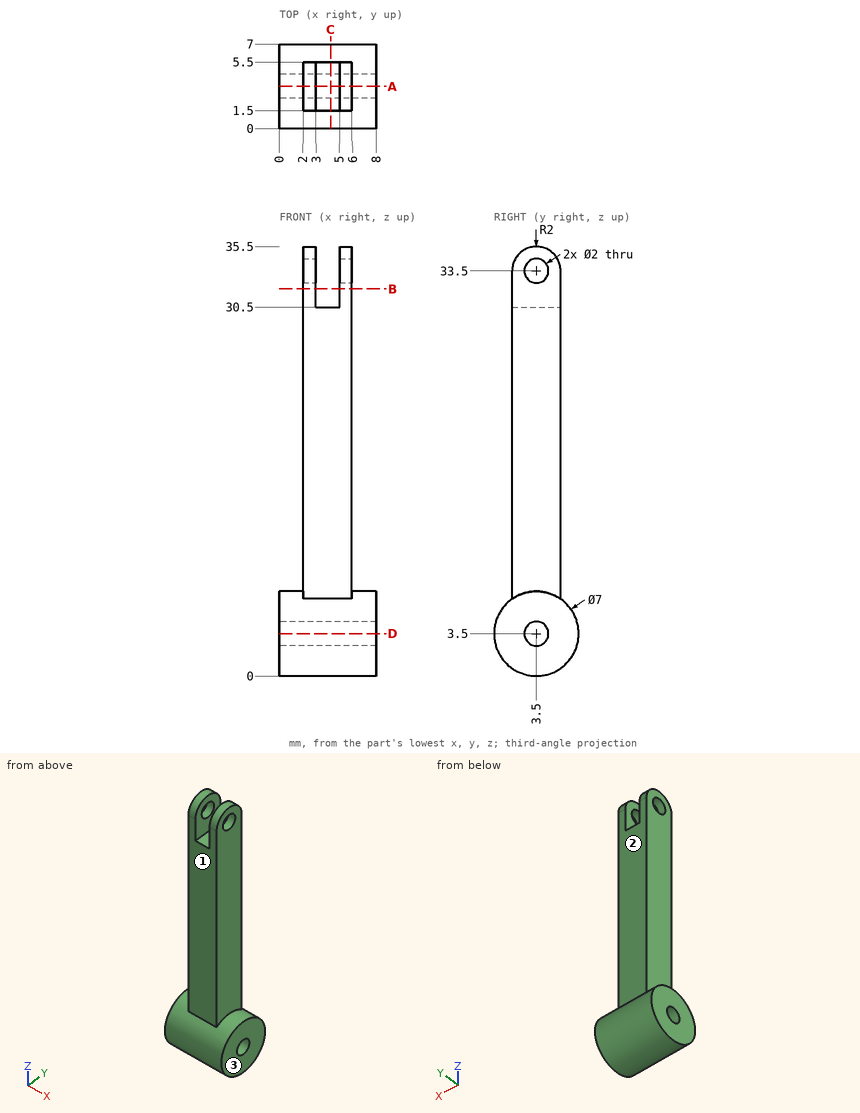
Study the drawing (mm; zero at the part's minimum x, y, z) and answer. A direction names the side the tool comes from. Give positions to 0.01 mm unless a question says otherwise; leave off trailing zeros. Write each loop counter-clockwise with the first axis right and the second up, starting at its lowest first coordinate (ties: lowest second). Pieces come first, ordered by that corner, then holes. Notation, with made-up numbers: (42, 1.25) -> (100, 1.25) arc R10 cw to (100, 20.25) -> close; hole circle Ø5 at (22, 38.5). An arc over 180 degrees is marked (long way). Write item = value, one per line.
Q1. Section B-B on z = 32 is taken. Determine the outline of the cut face in (x, y).
Computed values:
outline = (2, 1.5) -> (3, 1.5) -> (3, 5.5) -> (2, 5.5) -> close; (5, 1.5) -> (6, 1.5) -> (6, 5.5) -> (5, 5.5) -> close
Q2. Section C-C on x = 4.25 is taken. Determine the outline of the cut face in (y, z), and give its area (3 significant figures).
Computed values:
outline = (1.5, 6.37) arc R3.5 ccw (long way) to (5.5, 6.37) -> (5.5, 30.5) -> (1.5, 30.5) -> close; hole circle Ø2 at (3.5, 3.5)
area = 130 mm^2
Q3. Flat-ended cylindrical pins translate along their axes: pin 1 Ø1.8 at (y, z) = (3.5, 3.5) entering from +X; pin 2 Ø3 at (y, z) = (3, 27) entering from -X; pin 3 Ø3 at (x, z) = (5.5, 21.5) entering from -Y; pin 4 Ø4.5 at (x, z) = (3, 19) entering from +Y. Find the tip coordinate at first contact, or state that the pin passes through.
Computed values:
pin_1 = through
pin_2 = 2
pin_3 = 1.5
pin_4 = 5.5
Q4. Section D-D on z = 3.5 is taken. Determine the outline of the cut face in (x, y), and give its area (3 significant figures).
Computed values:
outline = (0, 0) -> (8, 0) -> (8, 2.5) -> (0, 2.5) -> close; (0, 4.5) -> (8, 4.5) -> (8, 7) -> (0, 7) -> close
area = 40.0 mm^2
Q5. Consider line 1 along Z through (x, y) = (5.55, 3.5); line 2 along Z through (x, y) = (4.75, 3.5); line 3 along X through (y, z) = (3, 9). Determine where each line is inside the solid, lowest interval first.
Computed values:
line_1 = 0 to 2.5, 4.5 to 32.5, 34.5 to 35.5
line_2 = 0 to 2.5, 4.5 to 30.5
line_3 = 2 to 6
Q6. A tool of negligible diameter and unlimited length cuts with its end or side. For the marked faces 1, 2 and 3, from which of +Z, -Z, +X, -X, +Y, -Y can it reach the whole face along a straight path? Write none if from no direction.
Computed values:
face_1 = +Z, +X, -X, -Y
face_2 = +Z, +X, -X, +Y
face_3 = +Z, -Z, +X, +Y, -Y
Q7. Section A-A on y = 3.5 is taken. Determine the outline of the cut face in (x, z).
Computed values:
outline = (0, 0) -> (8, 0) -> (8, 2.5) -> (0, 2.5) -> close; (0, 4.5) -> (8, 4.5) -> (8, 7) -> (6, 7) -> (6, 32.5) -> (5, 32.5) -> (5, 30.5) -> (3, 30.5) -> (3, 32.5) -> (2, 32.5) -> (2, 7) -> (0, 7) -> close; (2, 34.5) -> (3, 34.5) -> (3, 35.5) -> (2, 35.5) -> close; (5, 34.5) -> (6, 34.5) -> (6, 35.5) -> (5, 35.5) -> close
